Geometry: final body of the model. Coordinates: model frame, mm. A direction names the side the tool comes from. Round coordinates to 2 decimals unless told otherwise and drop trailing zeros. Order: outer loops, then holes, each group sorted by start corner. A loop starts at its lowest first (then second) coordinate and runs counter-clockwise, first axis right, second up. Notation, with made-up numbers: M 45,57 L 61,57 A32 cw 61,90 Z; hole C 49,-1.5 d2. An arc over 180 degrees is marked long. Return JSON: item names as keys, results as strings. Group by question number.
Q1. Mould query, pull axis X, two halves, no side actions, for faces 4 (the face through (-1.323, -0.208, -0.046)), 5 (the face through (44.83, -0.54, -2.44)), 6 (the face through (38.655, -0.434, -1.952)), 7 (the face through (-0.355, -0.434, 1.952)). Classes: released by +X, released by -X, zero draft, split by the parting line, or undercut.
Q2. Cut plane B-B on x = 34. Output: boundary loops of the cut face in (y, z), and give its area (3 significant figures).
Q3. Ray query, probe 1 along Z at (x, y) = (44.75, 0); probe 2 along X at (y, z) = (-1.55, 1.7). Return the intervals inside material, ascending.
Q4. Contact query for flat-ended pins moving along their axis: pin 1 (3 mm diameter, centred on x = 2.5, z = -0.5, fed in from +Y); pin 2 (2 mm diameter, centred on x = -4, z = -1.5, fed in from -Y); pin 3 (2 mm diameter, centred on y = 0, z = 0, fed in from +X); pin 4 (1.5 mm diameter, centred on y = -0.5, z = 0.5, fed in from -X). Output: stop coordinate, or through.
Q5. Access query for faces 1 (the face through (4, 0, 2.5)), 2 (the face through (45.396, 0.748, 0.976)), 3 (the face through (38.3, -2, 1)). Directions: +Z, -Z, +X, -X, +Y, -Y. A direction counts if a zero-diameter tool reaches every point of the face in a straight line with its end or side. Return the directions, or none.
Q6. Cut plane A-A on x = 44. Output: boundary loops of the cut face in (y, z).
Autodesk Inventor part; units mm, degrees
ref_plane "YZ Plane" through (0, 0, 0) normal (1, 0, 0) x (0, 1, 0)
ref_plane "XZ Plane" through (0, 0, 0) normal (0, 1, 0) x (-1, 0, 0)
ref_plane "XY Plane" through (0, 0, 0) normal (0, 0, 1) x (1, 0, 0)
sketch "Sketch_1" plane through (0, 0, 0) normal (0, 0, 1) x (1, 0, 0)
  line L0 (51, 0) -> (-12.7, 0)
  line L1 (-12.7, 0) -> (-12.7, 2)
  line L2 (-12.7, 2) -> (-12.2, 2.5)
  line L3 (-12.2, 2.5) -> (-0.2, 2.5)
  arc A0 (-0.2, 2.5) -> (0, 2.7) centre (-0.2, 2.7) ccw
  line L4 (0, 2.7) -> (0, 2.8)
  line L5 (0, 2.8) -> (0.2, 3)
  line L6 (0.2, 3) -> (38.1, 3)
  line L7 (38.1, 3) -> (38.3, 2.8)
  line L8 (38.3, 2.8) -> (38.3, 2.7)
  arc A1 (38.3, 2.7) -> (38.5, 2.5) centre (38.5, 2.7) ccw
  line L9 (38.5, 2.5) -> (50.5, 2.5)
  line L10 (50.5, 2.5) -> (51, 2)
  line L11 (51, 2) -> (51, 0)
  line L12 (51, 0) -> (-12.7, 0)
  line L13 (38.3, 2.7) -> (38.3, 2)
  line L14 (38.3, 2) -> (39, 2)
  line L15 (39, 2) -> (39, 2.5)
  line L16 (0, 2.7) -> (0, 2)
  line L17 (0, 2) -> (-0.7, 2)
  line L18 (-0.7, 2) -> (-0.7, 2.5)
  dimension "d17" = 0.7
  dimension "d18" = 2
  dimension "d20" = 0.7
  dimension "d21" = 2
revolve "Revolution1" add sketch "Sketch_1" angle 360 about axis through (51, 0, 0) along (1, 0, 0)
sketch "Sketch2" plane through (-12.7, 0, 0) normal (-1, 0, 0) x (0, 0, 1)
  point P0 (0, 0)
hole "Hole1" at (-12.7, 0, 0) direction (1, 0, 0) diameter 2.459 depth 10.7901 tip angle 120 countersink diameter 3 countersink angle 90
sketch "Sketch3" plane through (51, 0, 0) normal (1, 0, 0) x (0, 0, -1)
  point P0 (0, 0)
hole "Hole2" at (51, 0, 0) direction (-1, 0, 0) diameter 2.459 depth 10.7901 tip angle 120 countersink diameter 3 countersink angle 90
sketch "Sketch_28" plane through (0, 0, 0) normal (1, 0, 0) x (0, 0, -1)
  line L0 (-5, -6) -> (5, -6)
  line L1 (5, -6) -> (5, 3)
  line L2 (5, 3) -> (2.5, 3)
  line L3 (2.5, 3) -> (2.5, -3)
  line L4 (2.5, -3) -> (-2.5, -3)
  line L5 (-2.5, -3) -> (-2.5, 3)
  line L6 (-2.5, 3) -> (-5, 3)
  line L7 (-5, 3) -> (-5, -6)
extrude "Extrusion1" cut sketch "Sketch_28" along normal mid plane 16
revolve "回転2" cut sketch "Sketch_1" angle 360 about axis through (51, 0, 0) along (-1, 0, 0) contours L15 L14 L13 A1 L9 | L3 A0 L16 L17 L18
properties part number "SSFRMHHS6-38.3-F12.7-P5-T12.7-M3-SC0-TF12.7-TT12.7"
Result sheet:
{
 "1": {"face 4": "released by -X", "face 5": "zero draft", "face 6": "undercut", "face 7": "undercut"},
 "2": {"outline": "C 0,0 d6", "area": "28.3 mm²"},
 "3": {"probe 1": "z = -2.5 to -1.23, 1.23 to 2.5", "probe 2": "x = -12.4 to -0.7, 0 to 38.3, 39 to 50.7"},
 "4": {"pin 1": "stops at y = 3", "pin 2": "stops at y = -2.45", "pin 3": "stops at x = 40.08", "pin 4": "stops at x = -12.66"},
 "5": {"face 1": "+Z, -X, +Y, -Y", "face 2": "+X", "face 3": "none"},
 "6": {"outline": "C 0,0 d5; hole C 0,0 d2.46"}
}
